The listing builds one solid part. Answer for the finished solid, in the listing's coordinates (mm). Give positions to 0.01 mm unless a question says otherwise; leave off trailing zeros. Write each loop counter-clockwise with the first axis right and the second up, starting at its lowest first coordinate (ties: lowest second). Pieces come first, ordered by that corner, then holes. Notation, with made-up numbers: (31, 53) -> (62, 53) arc R27 cw to (62, 77) -> close; hole circle Ø7 at (34, 23). An arc over 180 degrees is marked (long way). Put each result on its own line as item: value. Start each with the question number.
1) A cutting plane is placed at D-D (x = -2.75). Write down the section's boundary in (y, z).
2) Flat-ended cylindrical pins translate along their axes: pin 1 Ø6 at (x, z) = (-9, -8) entering from +Y; pin 2 Ø0.5 at (x, y) = (-7, 0.5) entering from +Z. Find the tip coordinate at first contact, or state that the pin passes through.
3) A cutting plane is placed at B-B (y = 0.25). Write down the section's boundary in (x, z), then the cut area to 3 significant figures.
4) A cutting plane is placed at C-C (z = -14.5). Write down the section's boundary in (x, y), then the cut area to 3 significant figures.
5) A cutting plane is placed at A-A (x = 8.5). Write down the section's boundary in (y, z).
from build123d import *

# Parameters (mm, degrees)
BOSS_EXTRUDE1_DEPTH = 1


with BuildPart() as part:
    # Sketch1 → Boss-Extrude1 (new body)
    with BuildSketch(Plane(origin=(0, 0, 0), x_dir=(1, 0, 0), z_dir=(0, 1, 0))):
        Polygon((-12.726436998, 0), (12.726436998, 0), (12.726436998, 4.221634294), (2.211948406, 4.221634294), (2.211948406, 30.250890115), (-2.211948406, 30.250890115), (-11.390670326, 23.432410974), (-8.752594478, 19.881155024), (-2.211948406, 24.739920677), (-2.211948406, 4.221634294), (-12.726436998, 4.221634294), align=None)
        Polygon((-2.178869719, 30.150890115), (-11.250763541, 23.411768989), (-8.731952493, 20.021061809), (-2.111948406, 24.938779131), (-2.111948406, 4.121634294), (-12.626436998, 4.121634294), (-12.626436998, 0.1), (12.626436998, 0.1), (12.626436998, 4.121634294), (2.111948406, 4.121634294), (2.111948406, 30.150890115), align=None, mode=Mode.SUBTRACT)
    extrude(amount=BOSS_EXTRUDE1_DEPTH)


solid = part.part
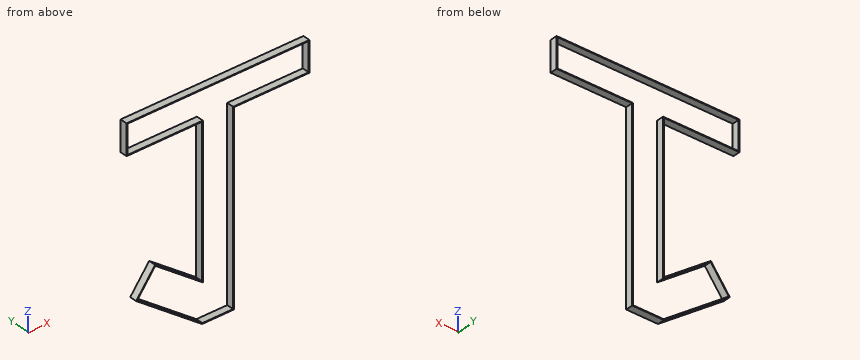
Reply:
1. outline: (0, -29.85) -> (1, -29.85) -> (1, -29.73) -> (0, -29.73) -> close; (0, -24.46) -> (1, -24.46) -> (1, -24.34) -> (0, -24.34) -> close; (0, -4.22) -> (1, -4.22) -> (1, -4.12) -> (0, -4.12) -> close; (0, -0.1) -> (1, -0.1) -> (1, 0) -> (0, 0) -> close
2. pin 1: passes through
2. pin 2: stops at z = 0
3. outline: (-12.73, -4.22) -> (-2.21, -4.22) -> (-2.21, -24.74) -> (-8.75, -19.88) -> (-11.39, -23.43) -> (-2.21, -30.25) -> (2.21, -30.25) -> (2.21, -4.22) -> (12.73, -4.22) -> (12.73, 0) -> (-12.73, 0) -> close; hole (-12.63, -4.12) -> (-2.11, -4.12) -> (-2.11, -24.94) -> (-8.73, -20.02) -> (-11.25, -23.41) -> (-2.18, -30.15) -> (2.11, -30.15) -> (2.11, -4.12) -> (12.63, -4.12) -> (12.63, -0.1) -> (-12.63, -0.1) -> close
3. area: 13.0 mm2
4. outline: (-2.21, 0) -> (-2.11, 0) -> (-2.11, 1) -> (-2.21, 1) -> close; (2.11, 0) -> (2.21, 0) -> (2.21, 1) -> (2.11, 1) -> close
4. area: 0.200 mm2
5. outline: (0, -4.22) -> (1, -4.22) -> (1, -4.12) -> (0, -4.12) -> close; (0, -0.1) -> (1, -0.1) -> (1, 0) -> (0, 0) -> close
